Design review of the part built by this model. Coordinates are the model's own, in mm. A direction names the side the tool comes from. Round coordinates to 2 decimals unless told otherwise and drop trailing zeros. Order: outer loops, then holes, each group sorted by start corner. A loop starts at its lowest first (then second) coordinate and runs counter-clockwise, first axis right, second up.
from build123d import *

# Parameters (mm, degrees)
F0_W     = 55
F0_H     = 50
F1_DEPTH = 10
F3_DEPTH = 35
F4_W     = 27.586387
F4_H     = 22.751658
F5_DEPTH = 15


with BuildPart() as f1:
    # F0 (on Top) → F1 (new body)
    with BuildSketch(Plane.XY):
        Rectangle(F0_W, F0_H)
    extrude(amount=F1_DEPTH)

    # F2 (on Top) → F3 (join)
    with BuildSketch(Plane.XY):
        Polygon((-27.396789, 24.932027), (-27.775984, 0), (0, 0), (0, 24.932027), align=None)
    extrude(amount=F3_DEPTH)

    # F4 (on Top) → F5 (join)
    with BuildSketch(Plane.XY):
        with Locations((13.793193, 13.935391)):
            Rectangle(F4_W, F4_H)
    extrude(amount=F5_DEPTH)


solid = f1.part
1) Take a section at A-A on x = -7.5. Give the boundary of the cut face in (y, z).
Results:
outline: (-25, 0) - (25, 0) - (25, 10) - (24.93, 10) - (24.93, 35) - (0, 35) - (0, 10) - (-25, 10) - close
2) Take a section at B-B on y = -15.5. Give the boundary of the cut face in (x, z).
Results:
outline: (-27.5, 0) - (27.5, 0) - (27.5, 10) - (-27.5, 10) - close
3) Clearance check with flat-ended pins moving along their axes: P1, Ø3, axis at x = 8, y = -13, coming from the +Z side; P2, Ø8, axis at y = -8, z = 5, coming from the -X side; P3, Ø3, axis at x = -12, z = 6.5, coming from the +Y side. State where each tip first meets the part, or that it passes through.
Results:
P1: stops at z = 10
P2: stops at x = -27.5
P3: stops at y = 25
4) To check wall thickness, follow line 1 along Y through (x, z) = (-23, 20.5); line 2 along Z through (x, y) = (-6.5, -23); line 3 along Y through (x, z) = (-10.5, 3). State the ranges of each line that lie inside material, in increasing order.
Results:
line 1: y = 0 to 24.93
line 2: z = 0 to 10
line 3: y = -25 to 25
5) Take a section at C-C on z = 18. Give the boundary of the cut face in (x, y).
Results:
outline: (-27.78, 0) - (0, 0) - (0, 24.93) - (-27.4, 24.93) - close
6) Take a section at D-D on x = 19.5. Give the boundary of the cut face in (y, z).
Results:
outline: (-25, 0) - (25.31, 0) - (25.31, 15) - (2.56, 15) - (2.56, 10) - (-25, 10) - close
7) For faces 1 (the face through (-14, 24.932, 22)), 2 (the face through (14, 14, 15)), 3 (the face through (-14, 25, 5)), list the 3-axis set-ups (+Z, -Z, +X, -X, +Y, -Y) from which the entire face can be reached by the end or side of a thin tool; tool diameter is ignored.
Results:
face 1: +Z, -X, +Y
face 2: +Z, +X, +Y, -Y
face 3: +Z, -Z, -X, +Y
